The listing builds one solid part. Answer for the finished solid, in the listing's coordinates (mm). Face numbers are marked on the shaded views. A direction names the side the tool comes from. Coordinates: 2 decimals unless noted, no trailing zeros. Order: outer loops, then holes, each group sorted by start corner. A loop starts at its lowest first (then second) coordinate and runs counter-clockwise, first axis right, second up. Notation, with made-up numbers: (-7, 63.25) - (33, 63.25) arc R26 ccw to (33, 99.25) - close; hole circle Ø8 at (17, 2). An arc over 180 degrees is marked (long way). Use a Markdown table: item, result. Add a question column.
Item 1: The part is cut by section D-D, the plane y = -14. Give the vertices of the cut face in (x, z), then the cut area to 3 significant figures.
Item 2: Find the intervals of material crossed by line 1 along X through (y, z) = (-11, 16); line 2 along Z through (x, y) = (-44.5, -17.5); line 3 along Y through (x, z) = (-48, 12.25), in increasing order.
Item 3: The part is cut by section A-A, the plane y = -10.25. Give the vertices of the cut face in (x, z), then the cut area to 3 significant figures.
Item 4: Flat-ended cylindrical pins translate along their axes: P1, Ø5, axis at x = -46.5, z = 9, coming from the +Y side; P2, Ø4, axis at y = -17.5, z = 13, coming from the -X side; P3, Ø5, axis at x = -60, y = -13, coming from the -Z side. Find the tip coordinate at first contact, or state that the pin passes through.
Item 5: The part is cut by section C-C, the plane z = 14.5. Give the vertices of the cut face in (x, y).
Item 6: For the marked faces 1, 2 and 3, determine the directions among +Z, -Z, +X, -X, +Y, -Y from which every point of the face is accessible in a straight line to the end or side of a thin tool.
from build123d import *

# Parameters (mm, degrees)
ESBO_O1_W                = 32.2
ESBO_O1_H                = 11.8
RESSALTO_EXTRUS_O1_DEPTH = 2
ESBO_O2_W                = 22.2
ESBO_O2_H                = 11.812594062
RESSALTO_EXTRUS_O2_DEPTH = 16
ESBO_O3_R                = 2.5
RESSALTO_EXTRUS_O3_DEPTH = 12


with BuildPart() as part:
    # Esboço1 → Ressalto-extrusão1 (new body)
    with BuildSketch(Plane.XY):
        with Locations((-49.254652801, -12.977504244)):
            Rectangle(ESBO_O1_W, ESBO_O1_H)
    extrude(amount=RESSALTO_EXTRUS_O1_DEPTH)

    # Esboço2 → Ressalto-extrusão2 (add)
    with BuildSketch(Plane.XY.offset(2)):
        with Locations((-49.254652801, -12.997877007)):
            Rectangle(ESBO_O2_W, ESBO_O2_H)
    extrude(amount=RESSALTO_EXTRUS_O2_DEPTH)

    # Esboço3 → Ressalto-extrusão3 (add)
    with BuildSketch(Plane(origin=(0, 0, 0), x_dir=(-1, 0, 0), z_dir=(0, 0, -1))):
        with Locations(Location((50.495961023, -13.245250528, 0), (0, 0, 180))):
            Circle(ESBO_O3_R)
    extrude(amount=RESSALTO_EXTRUS_O3_DEPTH)


solid = part.part
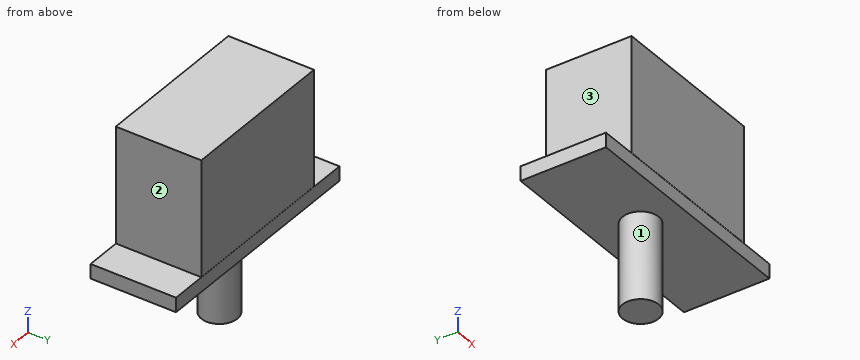
Solution:
| question | item | result |
|---|---|---|
| 1 | outline | (-65.35, 0) - (-52.88, 0) - (-52.88, -12) - (-48.11, -12) - (-48.11, 0) - (-33.15, 0) - (-33.15, 2) - (-38.15, 2) - (-38.15, 18) - (-60.35, 18) - (-60.35, 2) - (-65.35, 2) - close |
| 1 | area | 477 mm2 |
| 2 | line 1 | x = -60.35 to -38.15 |
| 2 | line 2 | z = 0 to 18 |
| 2 | line 3 | y = -18.9 to -7.09 |
| 3 | outline | (-65.35, 0) - (-33.15, 0) - (-33.15, 2) - (-38.15, 2) - (-38.15, 18) - (-60.35, 18) - (-60.35, 2) - (-65.35, 2) - close |
| 3 | area | 420 mm2 |
| 4 | P1 | stops at y = -7.09 |
| 4 | P2 | stops at x = -60.35 |
| 4 | P3 | stops at z = 0 |
| 5 | outline | (-60.35, -18.9) - (-38.15, -18.9) - (-38.15, -7.09) - (-60.35, -7.09) - close |
| 6 | face 1 | -Z |
| 6 | face 2 | +Z, +X, +Y, -Y |
| 6 | face 3 | +Z, -X, +Y, -Y |
